For this review, use the dimensioned drawing (mm, ordinates from the lowest corner) and the shaded views. A direction names the side the tool comes from. Round coordinates to 2 decimals unless told otherwise and drop trailing zeros. Write each loop counter-clockwise with the first axis right and the second up, starting at its lowest first coordinate (ties: lowest second). Pieces come first, ordered by that corner, then holes. Notation, with made-up numbers: (24.5, 16) -> (67.5, 16) arc R12 ccw to (67.5, 30) -> close; hole circle Ø11 at (47.5, -15). An arc over 180 degrees is marked (long way). Answer in a Markdown table with one row per item. Add a question column.
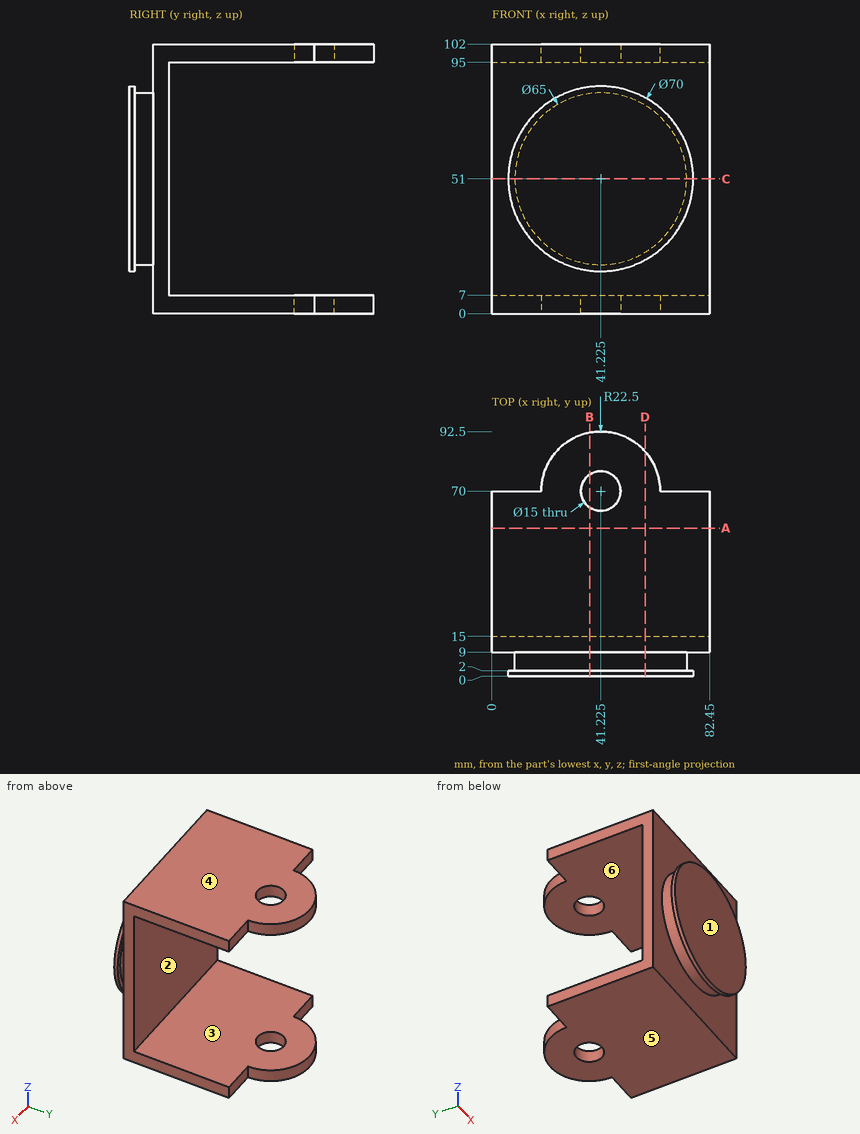
1. The part is to be moulded in two halves that separate along Z. For the marked faces 1, 2, 3 and 4, say which applies: pulls with the +Z half, pulls with the -Z half, needs draft (parallel to the pull), parting line crosses it, or undercut.
2. For L1, parallel to Z at x = 36, y = 47.5; L2, parallel to Y at x = 77.5, z = 66; L3, parallel to Y at x = 64, z = 68, list the stretches that pass through material, from the lowest coordinate up. Write a range as [from, to].
3. Clearance check with flat-ended pins moving along their axes: pin 1 Ø2 at (x, z) = (22.5, 69) entering from +Y; pin 2 Ø7.5 at (x, z) = (13, 2.5) entering from +Y. State where each tip first meets the part, or that it passes through.
4. Tool access review of the marked faces 5 and 6: name each direction out of +Z, -Z, +X, -X, +Y, -Y from which nothing blocks a thin tool from reaching the whole face with its end or side.
5. We need section C-C (z = 51). Write out the cut boundary in (x, y) (3 decimals).
6. We need section D-D (x = 58). Write out the cut boundary in (y, z).
7. We need section A-A (y = 56). Write out the cut boundary in (x, z), plus the area to 3 significant figures.
8. We need section B-B (x = 37). Write out the cut boundary in (y, z).
Response:
| question | item | result |
|---|---|---|
| 1 | face 1 | needs draft |
| 1 | face 2 | undercut |
| 1 | face 3 | undercut |
| 1 | face 4 | pulls with the +Z half |
| 2 | L1 | [0, 7], [95, 102] |
| 2 | L2 | [9, 15] |
| 2 | L3 | [0, 15] |
| 3 | pin 1 | y = 15 |
| 3 | pin 2 | y = 70 |
| 4 | face 5 | -Z, +X, -X, +Y, -Y |
| 4 | face 6 | +X, -X, +Y |
| 5 | outline | (0, 9) -> (8.725, 9) -> (8.725, 2) -> (6.225, 2) -> (6.225, 0) -> (76.225, 0) -> (76.225, 2) -> (73.725, 2) -> (73.725, 9) -> (82.45, 9) -> (82.45, 15) -> (0, 15) -> close |
| 6 | outline | (0, 20.28) -> (2, 20.28) -> (2, 23.16) -> (9, 23.16) -> (9, 0) -> (84.99, 0) -> (84.99, 7) -> (15, 7) -> (15, 95) -> (84.99, 95) -> (84.99, 102) -> (9, 102) -> (9, 78.84) -> (2, 78.84) -> (2, 81.72) -> (0, 81.72) -> close |
| 7 | outline | (0, 0) -> (82.45, 0) -> (82.45, 7) -> (0, 7) -> close; (0, 95) -> (82.45, 95) -> (82.45, 102) -> (0, 102) -> close |
| 7 | area | 1,150 mm2 |
| 8 | outline | (0, 16.26) -> (2, 16.26) -> (2, 18.78) -> (9, 18.78) -> (9, 0) -> (63.8, 0) -> (63.8, 7) -> (15, 7) -> (15, 95) -> (63.8, 95) -> (63.8, 102) -> (9, 102) -> (9, 83.22) -> (2, 83.22) -> (2, 85.74) -> (0, 85.74) -> close; (76.2, 0) -> (92.1, 0) -> (92.1, 7) -> (76.2, 7) -> close; (76.2, 95) -> (92.1, 95) -> (92.1, 102) -> (76.2, 102) -> close |
